Input: part model. Units: mm. Frame: model coordinates. Face numbers are marked on the shaded views. A direction names the side the tool comes from. Coordinates: 2 decimals unless noted, no trailing zeros. Loops run counter-clockwise (first coordinate to the right, second up) from the corner with the lowest first, then second, coordinate; pieces in that order, holes last. Notation, with made-up numbers: (24.5, 68.25) -> (63.5, 68.25) arc R19 ccw to (63.5, 87.25) -> close; hole circle Ø1 at (-36, 41). An arc over 180 degrees is marked (long way). Answer as a JSON object with one key per item and string values.
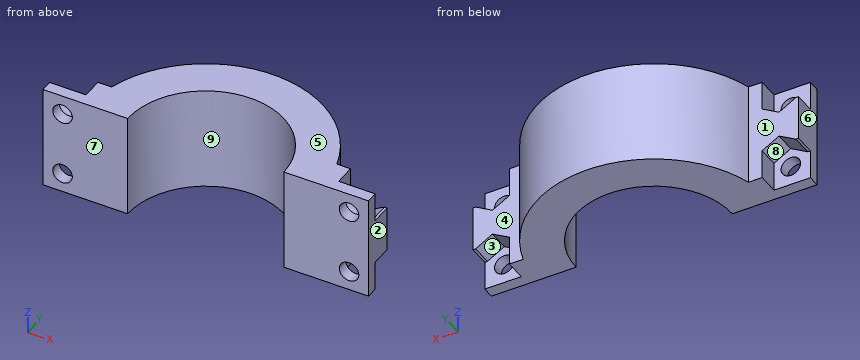
from build123d import *
from OCP.BRepAlgoAPI import BRepAlgoAPI_Cut
from OCP.TopTools import TopTools_ListOfShape

# Parameters (mm, degrees)
BOSS_EXTRUDE1_DEPTH = 16
CUT_EXTRUDE12_START = -22.166013
CUT_EXTRUDE12_DEPTH = 3.2
SKETCH14_R          = 1.5
CUT_EXTRUDE13_DEPTH = 50


with BuildPart() as part:
    # Sketch7 → Boss-Extrude1 (new body)
    with BuildSketch(Plane.XY):
        with BuildLine():
            Line((28.868798372, -27.16601268), (28.868798372, -22.16601268))
            Line((28.868798372, -22.16601268), (21.160414837, -22.16601268))
            ThreePointArc((21.160414837, -22.16601268), (3.868798372, -9.16601268), (-13.422818094, -22.16601268))
            Line((-13.422818094, -22.16601268), (-21.131201628, -22.16601268))
            Line((-21.131201628, -22.16601268), (-21.131201628, -27.16601268))
            Line((-21.131201628, -27.16601268), (-8.131201628, -27.16601268))
            ThreePointArc((-8.131201628, -27.16601268), (3.868798372, -15.16601268), (15.868798372, -27.16601268))
            Line((15.868798372, -27.16601268), (28.868798372, -27.16601268))
        make_face()
    extrude(amount=BOSS_EXTRUDE1_DEPTH)


with BuildPart() as cut_extrude12_tool:
    # Sketch13 → Cut-Extrude12 (new body)
    with BuildSketch(Plane(origin=(0, 0, 0), x_dir=(1, 0, 0), z_dir=(0, 1, 0)).offset(CUT_EXTRUDE12_START)):
        Polygon((-15.533125417, -4.5), (-15.533125417, -1.5), (-15.533125417, 0), (-18.131201628, 0), (-20.72927784, 0), (-21.131201628, 0), (-21.131201628, -4.5), (-20.72927784, -4.5), (-18.131201628, -6), align=None)
        Polygon((-21.131201628, -11.5), (-20.72927784, -11.5), (-18.131201628, -10), (-15.533125417, -11.5), (-15.533125417, -11.544775658), (-15.533125417, -16), (-18.131201628, -16), (-20.72927784, -16), (-21.131201628, -16), align=None)
        Polygon((23.27072216, -4.5), (23.27072216, -1.5), (23.27072216, 0), (25.868798372, 0), (28.466874583, 0), (28.868798372, 0), (28.868798372, -4.5), (28.466874583, -4.5), (25.868798372, -6), align=None)
        Polygon((28.466874583, -11.506491479), (25.868798372, -10.006491479), (23.27072216, -11.506491479), (23.27072216, -14.506491479), (23.27072216, -16.006491479), (25.868798372, -16.006491479), (28.466874583, -16.006491479), (28.868798372, -16.006491479), (28.868798372, -11.506491479), align=None)
    extrude(amount=-CUT_EXTRUDE12_DEPTH)


with BuildPart() as part_1:
    add(part.part)

    # Cut-Extrude12: cut by cut_extrude12_tool, with a tolerance
    cut_extrude12_stock = TopTools_ListOfShape()
    cut_extrude12_stock.Append(part_1.part.wrapped)
    cut_extrude12_tools = TopTools_ListOfShape()
    cut_extrude12_tools.Append(cut_extrude12_tool.part.wrapped)
    cut_extrude12_cut = BRepAlgoAPI_Cut()
    cut_extrude12_cut.SetArguments(cut_extrude12_stock)
    cut_extrude12_cut.SetTools(cut_extrude12_tools)
    cut_extrude12_cut.SetFuzzyValue(0.00001)
    cut_extrude12_cut.Build()
    add(Compound.cast(cut_extrude12_cut.Shape()).solids(), mode=Mode.REPLACE)

    # Sketch14 → Cut-Extrude13 (cut)
    with BuildSketch(Plane(origin=(0, 0, 0), x_dir=(1, 0, 0), z_dir=(0, 1, 0))):
        with Locations(Location((-18.131201628, -3, 0), (0, 0, 270))):
            Circle(SKETCH14_R)
        with Locations(Location((-18.131201628, -13, 0), (0, 0, 270))):
            Circle(SKETCH14_R)
        with Locations(Location((25.868798372, -3, 0), (0, 0, 270))):
            Circle(SKETCH14_R)
        with Locations(Location((25.868798372, -13, 0), (0, 0, 270))):
            Circle(SKETCH14_R)
    extrude(amount=-CUT_EXTRUDE13_DEPTH, mode=Mode.SUBTRACT)


solid = part_1.part
1. Section query A-A (y = -19). Return loops of the section in (x, z).
Reply:
{"outline": "(-12.17, 0) -> (-4.92, 0) -> (-4.92, 16) -> (-12.17, 16) -> close; (12.66, 0) -> (19.91, 0) -> (19.91, 16) -> (12.66, 16) -> close"}
2. Section query C-C (y = -21). Return loops of the section in (x, z).
Reply:
{"outline": "(-13.04, 0) -> (-6.43, 0) -> (-6.43, 16) -> (-13.04, 16) -> close; (14.16, 0) -> (20.78, 0) -> (20.78, 16) -> (14.16, 16) -> close"}
3. Access query for the marked faces 1, 2, 3, 4 and 5. Directions: +Z, -Z, +X, -X, +Y, -Y. A direction counts if a zero-diameter tool reaches every point of the face in a straight line with its end or side. Return the directions, or none.
Reply:
{"face 1": "+Z, -Z, -X, +Y", "face 2": "+Z, -Z, +X, +Y, -Y", "face 3": "-Z, +Y", "face 4": "+Z, -Z, +X, +Y", "face 5": "+Z, +X, -X, +Y, -Y"}
4. Pin query (flat end, axial travel): P1, Ø4, axis at x = 25.87, z = 13, coming from the -Y side; P2, Ø8, axis at x = 22, z = 13.5, coming from the +Y side; P3, Ø5, axis at x = -18.13, z = 3, coming from the +Y side; P4, Ø6, axis at x = 24.5, z = 8, coming from the +Y side. Return the tip coordinate at first contact, or that it passes through.
Reply:
{"P1": "stops at y = -27.17", "P2": "stops at y = -16.02", "P3": "stops at y = -25.37", "P4": "stops at y = -22.17"}
5. Section query B-B (z = 13). Return loops of the section in (x, y).
Reply:
{"outline": "(-21.13, -27.17) -> (-19.63, -27.17) -> (-19.63, -25.37) -> (-21.13, -25.37) -> close; (-16.63, -27.17) -> (-8.13, -27.17) arc R12 cw to (15.87, -27.17) -> (24.37, -27.17) -> (24.37, -25.37) -> (23.27, -25.37) -> (23.27, -22.17) -> (21.16, -22.17) arc R18 ccw to (-13.42, -22.17) -> (-15.53, -22.17) -> (-15.53, -25.37) -> (-16.63, -25.37) -> close; (27.37, -27.17) -> (28.87, -27.17) -> (28.87, -25.37) -> (27.37, -25.37) -> close"}
6. Line query: line 1 along X through (y, z) = (-26.4, 13); line 2 along X through (y, z) = (-26.6, 13); line 3 along X through (y, z) = (-22.75, 2.75). Output: solid intervals per line, ascending.
Reply:
{"line 1": "x = -21.13 to -19.63, -16.63 to -8.11, 15.84 to 24.37, 27.37 to 28.87", "line 2": "x = -21.13 to -19.63, -16.63 to -8.12, 15.86 to 24.37, 27.37 to 28.87", "line 3": "x = -15.53 to -7.29, 15.03 to 23.27"}
7. Mould query, pull axis X, two halves, no side actions, for the marked faces 6, 7, 8 and 9. Classes: pulls with the +X half, pulls with the -X half, needs draft (parallel to the pull), parting line crosses it, or undercut.
Reply:
{"face 6": "pulls with the -X half", "face 7": "needs draft", "face 8": "undercut", "face 9": "undercut"}
8. Section query D-D (z = 2). Return loops of the section in (x, y), plus the area to 3 significant figures.
Reply:
{"outline": "(-21.13, -27.17) -> (-19.25, -27.17) -> (-19.25, -25.37) -> (-21.13, -25.37) -> close; (-17.01, -27.17) -> (-8.13, -27.17) arc R12 cw to (15.87, -27.17) -> (24.75, -27.17) -> (24.75, -25.37) -> (23.27, -25.37) -> (23.27, -22.17) -> (21.16, -22.17) arc R18 ccw to (-13.42, -22.17) -> (-15.53, -22.17) -> (-15.53, -25.37) -> (-17.01, -25.37) -> close; (26.99, -27.17) -> (28.87, -27.17) -> (28.87, -25.37) -> (26.99, -25.37) -> close", "area": "311 mm2"}
